from build123d import *

# Parameters (mm, degrees)
BOSS_EXTRUDE1_DEPTH = 20
FILLET4_R           = 8
SHELL4_T            = -2
BOSS_EXTRUDE3_DEPTH = 2
FILLET5_R           = 3
SKETCH4_R           = 3
BOSS_EXTRUDE4_DEPTH = 5


with BuildPart() as part:
    # Sketch1 → Boss-Extrude1 (new body)
    with BuildSketch(Plane(origin=(0, 0, 0), x_dir=(1, 0, 0), z_dir=(0, 1, 0))):
        with BuildLine():
            Line((-30.483789425, 33.101942273), (-50.483789425, 40.943705319))
            ThreePointArc((-50.483789425, 40.943705319), (-64.988970557, 1.197374595), (-51.957731338, -39.056294681))
            ThreePointArc((-51.957731338, -39.056294681), (-37.955573489, -41.04113109), (-35.97073708, -27.038973241))
            ThreePointArc((-35.97073708, -27.038973241), (-44.813875675, 4.088587411), (-30.483789425, 33.101942273))
        make_face()
    extrude(amount=BOSS_EXTRUDE1_DEPTH)

    # Fillet4
    fillet4_edges = [part.edges().sort_by_distance(p)[0] for p in [
        (-44.813875675, 20, -4.088587411),
        (-64.988970557, 20, -1.197374595),
        (-44.813875675, 0, -4.088587411),
        (-37.955573489, 0, 41.04113109),
        (-64.988970557, 0, -1.197374595),
        (-37.955573489, 20, 41.04113109),
    ]]
    fillet(fillet4_edges, radius=FILLET4_R)

    # Shell4
    shell4_openings = [part.faces().sort_by_distance(p)[0] for p in [
        (-40.508625428, 10, -37.032561699),
    ]]
    offset(amount=SHELL4_T, openings=shell4_openings, kind=Kind.INTERSECTION)

    # Sketch2 → Boss-Extrude3 (add)
    with BuildSketch(Plane(origin=(0, 20, 0), x_dir=(1, 0, 0), z_dir=(0, 1, 0))):
        Polygon((-39.36151224, 36.582792208), (-62.636385717, 45.708594344), (-69.937027426, 27.088695563), (-51.317128644, 19.788053854), align=None)
    extrude(amount=-BOSS_EXTRUDE3_DEPTH)

    # Fillet5
    fillet5_edges = [part.edges().sort_by_distance(p)[0] for p in [
        (-53.682873098, 18, -31.597158652),
    ]]
    fillet(fillet5_edges, radius=FILLET5_R)

    # Sketch4 → Boss-Extrude4 (add)
    with BuildSketch(Plane.XZ.offset(-18)):
        with Locations(Location((-59.806571448, -39.228459222, 0), (0, 0, 90))):
            Circle(SKETCH4_R)
        with Locations(Location((-63.456892303, -29.918509831, 0), (0, 0, 55.543794566))):
            Circle(SKETCH4_R)
    extrude(amount=BOSS_EXTRUDE4_DEPTH)


solid = part.part
Design review of the part built by this model. Coordinates are the model's own, in mm. A direction names the side the tool comes from. Round coordinates to 2 decimals unless told otherwise and drop trailing zeros.
1) Draft analysis for pull direction Y (two halves, no side actions). For faces 4 (the flat face through (-62.838, 18.613, -24.305)), 5 (the flat face through (-62, 18, -35)), 6 (the flat face through (-53.3, 2, -1.6)), state which applies: released by +Y, released by -Y, zero draft, split by the parting line, or undercut.
The answers:
face 4: zero draft
face 5: released by -Y
face 6: undercut
2) Machinability: for faces 1 (the cylindrical face through (-46.883, 9.972, -3.312)), 2 (the cylindrical face through (-60.708, 15.535, -36.367)), 3 (the flat face through (-60, 13, -39)), which of the approach directions +Z, -Z, +X, -X, +Y, -Y give a long, thin tool a straight path to every point of the face, cutting with its end or side? Answer none if there is none.
The answers:
face 1: none
face 2: -Y
face 3: -Z, -X, -Y
3) Clearance check with flat-ended pins moving along their axes: pin 1 Ø8.5 at (x, z) = (-61.5, -36) entering from -Y; pin 2 Ø3 at (y, z) = (16, -9.5) entering from +X; pin 3 Ø1.5 at (y, z) = (14, 17) entering from -X. State where each tip first meets the part, or that it passes through.
The answers:
pin 1: stops at y = 13
pin 2: stops at x = -44.3
pin 3: stops at x = -62.74
4) Consider section A-A (x = -44). Count the separate pieces of the cut face and the enclosed holes in it, plus the area to 3 significant figures.
The answers:
separate pieces: 2
enclosed holes: 1
area: 396 mm2
5) For L1, parallel to Y at x = -53.5, z = -8.5; L2, parallel to Z at x = -52, y = 14.25; L3, parallel to Z at x = -50, y = 6, list the stretches that pass through material, from the lowest coordinate up.
The answers:
L1: y = 0 to 2, 18 to 20
L2: z = -38.46 to -34.79, 34.79 to 38.46
L3: z = -40.75 to -37.76, 37.76 to 40.7
